Check sheet for the modelled part. Datum: model origin and axes. Units: mm. A direction names the side the tool comes from. Coordinates: 2 decimals unless noted, no trailing zeros. Loops run counter-clockwise (first coordinate to the right, second up) from the corner with the lowest first, then second, coordinate; pieces in that order, holes last. Notation, with made-up numbers: M 36.5,-28.5 L 50.5,-28.5 A22 cw 50.5,-2.5 Z; hole C -40,-39.75 d10. An arc over 180 degrees is marked long. Return JSON: item names as keys, results as strings.
from build123d import *

# Parameters (mm, degrees)
SKETCH1_R               = 4.77
SKETCH1_R_2             = 1.59
BOSS_EXTRUDE1_DEPTH     = 18
CHAMFER1_SIZE           = 2.22
CHAMFER1_SIZE_2         = 6.88
CHAMFER2_SIZE           = 6.88
CHAMFER2_SIZE_2         = 2.22
CUT_EXTRUDE1_DEPTH      = 35.136329621
CUT_EXTRUDE1_DEPTH_BACK = 35.136329621
SKETCH3_W               = 9
SKETCH3_H               = 9.53


with BuildPart() as part:
    # Sketch1 → Boss-Extrude1 (new body)
    with BuildSketch(Plane.XY):
        with BuildLine():
            Line((-27.31, 0), (-27.31, 5))
            Line((-27.31, 5), (-3.328977305, 9.185358464))
            ThreePointArc((-3.328977305, 9.185358464), (5.609313315, 7.999281476), (9.77, 0))
            Line((9.77, 0), (21.07, -4.844453369))
            Line((21.07, -4.844453369), (20.210354499, -9.77))
            Line((20.210354499, -9.77), (0, -9.77))
            ThreePointArc((0, -9.77), (-6.908433252, -6.908433252), (-9.77, 0))
            Line((-9.77, 0), (-27.31, 0))
        make_face()
        Circle(SKETCH1_R, mode=Mode.SUBTRACT)
        with Locations((-24.77, 2.5)):
            Circle(SKETCH1_R_2, mode=Mode.SUBTRACT)
        with Locations((18.055286128, -7.344453369)):
            Circle(SKETCH1_R_2, mode=Mode.SUBTRACT)
    extrude(amount=BOSS_EXTRUDE1_DEPTH)

    # Chamfer1
    # the kernel refuses this chamfer: 6.88, 2.22 mm, written as the material it takes off along each edge
    with BuildSketch(Plane(origin=(-27.31, -17.856007533, 18), x_dir=(-0.11292116623223689, 0, -0.9936039503830244), z_dir=(0, 1, 0))) as chamfer1_piece_1:
        Polygon((CHAMFER1_SIZE * 0.993603950383, -CHAMFER1_SIZE * 0.112921166232), (-CHAMFER1_SIZE_2 * 0.112921166232, -CHAMFER1_SIZE_2 * 0.993603950383), (0, 0), align=None)
    extrude(amount=40.712015065, mode=Mode.SUBTRACT)
    with BuildSketch(Plane(origin=(-27.31, -17.856007533, 0), x_dir=(-0.1129211662322369, 0, 0.9936039503830242), z_dir=(0, 1, 0))) as chamfer1_piece_2:
        Polygon((CHAMFER1_SIZE * 0.993603950383, CHAMFER1_SIZE * 0.112921166232), (-CHAMFER1_SIZE_2 * 0.112921166232, CHAMFER1_SIZE_2 * 0.993603950383), (0, 0), align=None)
    extrude(amount=40.712015065, mode=Mode.SUBTRACT)

    # Chamfer2
    # the kernel refuses this chamfer: 6.88, 2.22 mm, written as the material it takes off along each edge
    with BuildSketch(Plane(origin=(24.13996731, 12.745666179, 0), x_dir=(-0.9850403671370294, 0.1719170650041742, -0.011832069594835619), z_dir=(-0.17192910027940936, -0.985109326154774, 0))) as chamfer2_piece_1:
        Polygon((CHAMFER2_SIZE * 0.999929998614, -CHAMFER2_SIZE * 0.0118320695948), (-CHAMFER2_SIZE_2 * 0.0118320695948, -CHAMFER2_SIZE_2 * 0.999929998614), (0, 0), align=None)
    extrude(amount=40.712015065, mode=Mode.SUBTRACT)
    with BuildSketch(Plane(origin=(24.13996731, 12.745666179, 18), x_dir=(-0.9850403671370294, 0.1719170650041742, 0.011832069594835435), z_dir=(-0.17192910027940936, -0.985109326154774, 0))) as chamfer2_piece_2:
        Polygon((CHAMFER2_SIZE * 0.999929998614, CHAMFER2_SIZE * 0.0118320695948), (-CHAMFER2_SIZE_2 * 0.0118320695948, CHAMFER2_SIZE_2 * 0.999929998614), (0, 0), align=None)
    extrude(amount=40.712015065, mode=Mode.SUBTRACT)

    # Sketch3 → Cut-Extrude1 (cut, two sides: drawn at the far end of the back side and taken through both)
    with BuildSketch(Plane(origin=(0, 0, 0), x_dir=(1, 0, 0), z_dir=(0, 1, 0)).offset(-CUT_EXTRUDE1_DEPTH_BACK)):
        with Locations((-22.81, -9)):
            Rectangle(SKETCH3_W, SKETCH3_H)
        with BuildLine():
            Line((-9.31, -3.8), (0.89, -3.8))
            ThreePointArc((0.89, -3.8), (6.09, -9), (0.89, -14.2))
            Line((0.89, -14.2), (-9.31, -14.2))
            ThreePointArc((-9.31, -14.2), (-14.51, -9), (-9.31, -3.8))
        make_face()
        with Locations((16.57, -9)):
            Rectangle(SKETCH3_W, SKETCH3_H)
    extrude(amount=CUT_EXTRUDE1_DEPTH + CUT_EXTRUDE1_DEPTH_BACK, mode=Mode.SUBTRACT)


solid = part.part
1) Section check C-C on x = -1. Record the cut outline in (y, z), then the cut area to 3 significant figures.
Answers:
{"outline": "M -9.72,0 L -4.66,0 L -4.66,3.8 L -9.72,3.8 Z; M -9.72,14.2 L -4.66,14.2 L -4.66,18 L -9.72,18 Z; M 4.66,0 L 9.72,0 L 9.72,3.8 L 4.66,3.8 Z; M 4.66,14.2 L 9.72,14.2 L 9.72,18 L 4.66,18 Z", "area": "76.8 mm²"}
2) Draft check along Z on faces 5 (the face through (-23.154, 3.746, 17.121)), 6 (the face through (16, -6, 13.765)), 7 (the face through (8, -9.77, 9)), 8 (the face through (16.5, -6.31, 0.85)). Enter one of: +Z half, -Z half, draft (parallel to the pull), parting line (faces both ways), or undercut.
Answers:
{"face 5": "+Z half", "face 6": "undercut", "face 7": "draft", "face 8": "-Z half"}
3) Go/stop test with flat-tipped pins: pin 1 Ø7 at (y, z) = (3, 8.5) entering from -X; pin 2 Ø3 at (x, z) = (-14, 14) entering from +Y; pin 3 Ø3.5 at (x, y) = (-24.77, 2.5) entering from -Z. Record where each tip stops, or that it passes through.
Answers:
{"pin 1": "x = -18.31", "pin 2": "y = 7.58", "pin 3": "z = 0.84"}
4) Section check A-A on y = -3.5. Record the cut outline in (x, z) (3 decimals), then the cut area to 3 significant figures.
Answers:
{"outline": "M -9.122,0 L -3.241,0 L -3.241,3.8 L -9.122,3.8 Z; M -9.122,14.2 L -3.241,14.2 L -3.241,18 L -9.122,18 Z; M 3.241,0 L 14.321,0 L 17.934,1.149 L 17.934,4.235 L 12.07,4.235 L 12.07,13.765 L 17.934,13.765 L 17.934,16.851 L 14.321,18 L 3.241,18 L 3.241,13.638 A5.2 cw 3.241,4.362 Z", "area": "230 mm²"}
5) Section check B-B on z = 8.25. Record the cut outline in (x, y), then the cut area to 3 significant figures.
Answers:
{"outline": "M -18.31,0 L -14.46,0 L -14.46,7.24 L -18.31,6.57 Z; M 6.04,-9.77 L 12.07,-9.77 L 12.07,-0.99 L 9.77,0 A9.77 ccw 6.04,7.68 Z", "area": "104 mm²"}
6) Set-up check for faces 1 (the face through (-22, 3, 4.235)), 2 (the face through (-14.51, 3.75, 9.11)), 3 (the face through (12.07, -5, 9)), 4 (the face through (-23.154, 3.746, 0.879)): record each of +Z, -Z, +X, -X, +Y, -Y from which the full face is reachable in a straight line by a thin tool's end or side.
Answers:
{"face 1": "-X, +Y, -Y", "face 2": "+Y, -Y", "face 3": "+X, +Y, -Y", "face 4": "-Z, -X, +Y, -Y"}
7) Scan lines: line 1 along Z through (x, y) = (-4.5, 4.5); line 2 along Y through (x, z) = (0, 16); line 3 along Z through (x, y) = (-19.5, 6.25) (3 decimals). Record each from-to range of solid material in increasing order. Write a range as [from, to].
Answers:
{"line 1": "[0, 3.8], [14.2, 18]", "line 2": "[-9.77, -4.77], [4.77, 9.77]", "line 3": "[0, 4.235], [13.765, 18]"}
8) Section check D-D on y = 2.5. Record the cut outline in (x, z) (3 decimals), then the cut area to 3 significant figures.
Answers:
{"outline": "M -27.31,2.22 L -26.36,1.913 L -26.36,4.235 L -27.31,4.235 Z; M -27.31,13.765 L -26.36,13.765 L -26.36,16.087 L -27.31,15.78 Z; M -23.18,0.887 L -20.43,0 L -4.062,0 L -4.062,3.8 L -9.31,3.8 A5.2 cw -9.31,14.2 L -4.062,14.2 L -4.062,18 L -20.43,18 L -23.18,17.113 L -23.18,13.765 L -18.31,13.765 L -18.31,4.235 L -23.18,4.235 Z; M 4.062,0 L 9.445,0 L 9.445,18 L 4.062,18 L 4.062,13.12 A5.2 cw 4.062,4.88 Z", "area": "288 mm²"}
